Read the model definition and answer for the solid it produces. Units are mm, in the model's axes. A direction names the side the tool comes from. Give positions to 0.01 mm unless a question says otherwise; leave off trailing zeros. Loops run counter-clockwise (first coordinate to the right, second up) from the corner with the lowest first, then second, coordinate; pieces in that order, holes last. Notation, with made-up numbers: (28.25, 9) - (75.25, 9) arc R17 ccw to (75.25, 38) - close; hole circle Ø8 at (2.25, 28). An arc over 180 degrees is marked (long way). Use a Markdown table: item, result. Add a question column.
Item 1: A cutting plane is placed at C-C (x = -12.75). Determine the outline of the cut face in (y, z), plus the area to 3 significant figures.
Item 2: A cutting plane is placed at B-B (y = 15). Determine the outline of the cut face in (x, z).
Item 3: Consider probe 1 along Z at (x, y) = (-15, 12.75); probe 2 along Y at (x, z) = (20, -7.15); probe 3 along Y at (x, z) = (0, 5.55). Determine where each line is inside the solid, lowest interval first. Write a range as [from, to].
Item 4: For a pull along X with two mould halves and no side action, classify faces 6 (the face through (-24.57, 24.8, -6.32)), 7 (the face through (0, 13, -7.8)), 8 (the face through (22, 1, 0)) as +X half, -X half, draft (parallel to the pull), parting line (faces both ways), or undercut.
Item 5: Which of the six approach directions +Z, -Z, +X, -X, +Y, -Y give full straight-line access (tool end or side, diameter ignored) to faces 1 (the face through (0.208, 21.336, 6.279)), 2 (the face through (-24.57, 24.8, 6.32)), 3 (the face through (17.93, 3.65, 0.65)), 4 (the face through (-6, 2.1, -2)), 5 (the face through (-20.234, 23.535, -6.279))?
Item 6: A cutting plane is placed at A-A (z = -6.5). Determine the outline of the cut face in (x, y), plus the area to 3 significant figures.
Item 7: A cutting plane is placed at D-D (x = 19.5). Determine the outline of the cut face in (y, z), plus the area to 3 significant figures.
Item 8: Each of these flat-tipped pins is pushed along its axis until it touches: P1, Ø2.5, axis at x = 4.5, z = 0, coming from the -Y side; P2, Ø4, axis at x = 19.5, z = 0, coming from the +Y side. Where does it stop, or does it pass through?
from build123d import *

# Parameters (mm, degrees)
SKETCH1_W                = 50
SKETCH1_H                = 9.6
BOSS_EXTRUDE1_DEPTH      = 5.25
SKETCH2_R                = 2.5
CUT_EXTRUDE1_DEPTH       = 2.1
M3_CLEARANCE_HOLE1_D     = 3.4
M3_CLEARANCE_HOLE1_DEPTH = 7.978536948
M3_CLEARANCE_HOLE1_TIP   = 1.021463052
SKETCH5_W                = 50
SKETCH5_H                = 25.25
BOSS_EXTRUDE2_DEPTH      = 3
FILLET1_R                = 1.5
M3_CLEARANCE_HOLE4_D     = 3.2
M3_CLEARANCE_HOLE4_DEPTH = 3.03862301
M3_CLEARANCE_HOLE4_TIP   = 0.96137699
M3_CLEARANCE_HOLE5_D     = 3.6
M3_CLEARANCE_HOLE5_DEPTH = 3.918450886
M3_CLEARANCE_HOLE5_TIP   = 1.081549114
FILLET2_R                = 1.5


with BuildPart() as part:
    # Sketch1 → Boss-Extrude1 (new body)
    with BuildSketch(Plane(origin=(0, 0, 0), x_dir=(1, 0, 0), z_dir=(0, 1, 0))):
        Rectangle(SKETCH1_W, SKETCH1_H)
    extrude(amount=BOSS_EXTRUDE1_DEPTH)

    # Sketch2 → Cut-Extrude1 (cut)
    with BuildSketch(Plane.XZ):
        with Locations(Location((-19.5, 0, 0), (0, 0, 270))):
            Circle(SKETCH2_R)
        with Locations(Location((-5.5, 0, 0), (0, 0, 270))):
            Circle(SKETCH2_R)
        with Locations(Location((5.5, 0, 0), (0, 0, 270))):
            Circle(SKETCH2_R)
        with Locations(Location((19.5, 0, 0), (0, 0, 270))):
            Circle(SKETCH2_R)
    extrude(amount=-CUT_EXTRUDE1_DEPTH, mode=Mode.SUBTRACT)

    # M3 Clearance Hole1
    with Locations(Plane(origin=(0, 5.25, 0), x_dir=(1, 0, 0), z_dir=(0, 1, 0))):
        with Locations((-19.5, 0), (-5.5, 0), (5.5, 0), (19.5, 0)):
            Hole(M3_CLEARANCE_HOLE1_D / 2, depth=M3_CLEARANCE_HOLE1_DEPTH)
            with Locations((0, 0, -(M3_CLEARANCE_HOLE1_DEPTH + M3_CLEARANCE_HOLE1_TIP / 2))):  # 118° drill point
                Cone(0, M3_CLEARANCE_HOLE1_D / 2, M3_CLEARANCE_HOLE1_TIP, mode=Mode.SUBTRACT)

    # Sketch5 → Boss-Extrude2 (add)
    with BuildSketch(Plane.XY.offset(4.8)):
        with Locations((0, 12.625)):
            Rectangle(SKETCH5_W, SKETCH5_H)
    boss_extrude2 = extrude(amount=BOSS_EXTRUDE2_DEPTH)

    # Mirror1: Boss-Extrude2 across plane
    add(boss_extrude2.mirror(Plane.XY))

    # Fillet1
    fillet1_edges = [part.edges().sort_by_distance(p)[0] for p in [
        (0, 5.25, 4.8),
        (0, 5.25, -4.8),
    ]]
    fillet(fillet1_edges, radius=FILLET1_R)

    # M3 Clearance Hole4
    with Locations(Plane.XY.offset(7.8)):
        with Locations((0, 19.75)):
            Hole(M3_CLEARANCE_HOLE4_D / 2, depth=M3_CLEARANCE_HOLE4_DEPTH)
            with Locations((0, 0, -(M3_CLEARANCE_HOLE4_DEPTH + M3_CLEARANCE_HOLE4_TIP / 2))):  # 118° drill point
                Cone(0, M3_CLEARANCE_HOLE4_D / 2, M3_CLEARANCE_HOLE4_TIP, mode=Mode.SUBTRACT)

    # M3 Clearance Hole5
    with Locations(Plane(origin=(0, 0, -7.8), x_dir=(-1, 0, 0), z_dir=(0, 0, -1))):
        with Locations((-20, 21.75), (20, 21.75), (12.75, 11.75), (-12.75, 11.75)):
            Hole(M3_CLEARANCE_HOLE5_D / 2, depth=M3_CLEARANCE_HOLE5_DEPTH)
            with Locations((0, 0, -(M3_CLEARANCE_HOLE5_DEPTH + M3_CLEARANCE_HOLE5_TIP / 2))):  # 118° drill point
                Cone(0, M3_CLEARANCE_HOLE5_D / 2, M3_CLEARANCE_HOLE5_TIP, mode=Mode.SUBTRACT)

    # Fillet2
    fillet2_edges = [part.edges().sort_by_distance(p)[0] for p in [
        (-25, 25.25, 6.3),
        (25, 25.25, 6.3),
        (-25, 25.25, -6.3),
        (25, 25.25, -6.3),
    ]]
    fillet(fillet2_edges, radius=FILLET2_R)


solid = part.part
Geometry says:
| question | item | result |
|---|---|---|
| 1 | outline | (0, -7.8) - (9.95, -7.8) - (9.95, -4.8) - (6.75, -4.8) arc R1.5 cw to (5.25, -3.3) - (5.25, 3.3) arc R1.5 cw to (6.75, 4.8) - (25.25, 4.8) - (25.25, 7.8) - (0, 7.8) - close; (13.55, -7.8) - (25.25, -7.8) - (25.25, -4.8) - (13.55, -4.8) - close |
| 1 | area | 192 mm² |
| 2 | outline | (-25, -7.8) - (25, -7.8) - (25, -4.8) - (-25, -4.8) - close; (-25, 4.8) - (25, 4.8) - (25, 7.8) - (-25, 7.8) - close |
| 3 | probe 1 | [-7.8, -4.8], [4.8, 7.8] |
| 3 | probe 2 | [0, 19.95], [23.55, 25.25] |
| 3 | probe 3 | [0, 18.15], [21.35, 25.25] |
| 4 | face 6 | -X half |
| 4 | face 7 | draft |
| 4 | face 8 | undercut |
| 5 | face 1 | +Z |
| 5 | face 2 | +Z, -Z, -X, +Y |
| 5 | face 3 | +Y, -Y |
| 5 | face 4 | -Y |
| 5 | face 5 | -Z |
| 6 | outline | (-25, 0) - (25, 0) - (25, 23.75) arc R1.5 ccw to (23.5, 25.25) - (-23.5, 25.25) arc R1.5 ccw to (-25, 23.75) - close; hole circle Ø3.6 at (-20, 21.75); hole circle Ø3.6 at (-12.75, 11.75); hole circle Ø3.6 at (12.75, 11.75); hole circle Ø3.6 at (20, 21.75) |
| 6 | area | 1,220 mm² |
| 7 | outline | (0, -7.8) - (20.02, -7.8) - (20.02, -4.8) - (6.75, -4.8) arc R1.5 cw to (5.25, -3.3) - (5.25, -1.7) - (2.1, -1.7) - (2.1, -2.5) - (0, -2.5) - close; (0, 2.5) - (2.1, 2.5) - (2.1, 1.7) - (5.25, 1.7) - (5.25, 3.3) arc R1.5 cw to (6.75, 4.8) - (25.25, 4.8) - (25.25, 7.8) - (0, 7.8) - close; (23.48, -7.8) - (25.25, -7.8) - (25.25, -4.8) - (23.48, -4.8) - close |
| 7 | area | 171 mm² |
| 8 | P1 | y = 2.1 |
| 8 | P2 | y = 5.25 |
